```python
from build123d import *

# Parameters (mm, degrees)
SZKIC1_W                    = 100
SZKIC1_H                    = 60
SZKIC1_R                    = 10
DODANIE_WYCI_GNI_CIE1_DEPTH = 15
DODANIE_WYCI_GNI_CIE2_DEPTH = 15
SZKIC3_R                    = 6.5
DODANIE_WYCI_GNI_CIE5_DEPTH = 15


with BuildPart() as part:
    # Szkic1 → Dodanie-wyci_gni_cie1 (new body)
    with BuildSketch(Plane.XY):
        Rectangle(SZKIC1_W, SZKIC1_H)
        Circle(SZKIC1_R, mode=Mode.SUBTRACT)
    extrude(amount=-DODANIE_WYCI_GNI_CIE1_DEPTH)



with BuildPart() as body_2:
    # Szkic2 → Dodanie-wyci_gni_cie2 (new body)
    with BuildSketch(Plane.XY.offset(37)):
        Polygon((-50, 30), (-50, 15), (25, 15), (25, -30), (50, -30), (50, 30), align=None)
    extrude(amount=DODANIE_WYCI_GNI_CIE2_DEPTH)


with BuildPart() as part_1:
    add(part.part)

    add(body_2.part)  # Dodanie-wyci_gni_cie5 merges body 2
    # Szkic3 → Dodanie-wyci_gni_cie5 (add)
    with BuildSketch(Plane(origin=(0, -30, 0), x_dir=(-1, 0, 0), z_dir=(0, -1, 0))):
        Polygon((-25, 0), (-25, -37), (-50, -37), (-50, -15), (-75, -15), (-75, 15), (-50, 15), (-50, 0), align=None)
        with Locations(Location((-63, 0, 0), (0, 0, 90))):
            Circle(SZKIC3_R, mode=Mode.SUBTRACT)
    extrude(amount=-DODANIE_WYCI_GNI_CIE5_DEPTH)


solid = part_1.part
```
Part model, mm, in its own coordinate system. A direction names the side the tool comes from. Round coordinates to 2 decimals unless told otherwise and drop trailing zeros. Order: outer loops, then holes, each group sorted by start corner. A loop starts at its lowest first (then second) coordinate and runs counter-clockwise, first axis right, second up. Notation, with made-up numbers: M 12,-15 L 21,-15 A16 ccw 21,7 Z; hole C -19,-31.5 d11. An arc over 180 degrees is marked long. Answer in a Markdown table with one row per item. Add a question column.
Q1. Wall check: L1, parallel to Z at x = -39, y = 21; L2, parallel to X at y = 9, z = 45; L3, parallel to Y at x = 64, z = 12.5. Give the ranges that are in metal, low to high. Write a range as from..to.
Q2. Mould opens along Z. For faces 6 (the face through (13, 0, -15)), 7 (the face through (1, 30, 44)), 8 (the face through (50, -15, 11)) say: +Z half, -Z half, draft (parallel to the pull), parting line (faces both ways), or undercut.
Q3. Cut at D-D on x = 0. Give the cut face in (y, z), and give its area (3 significant figures).
Q4. Pin check, flat tips, straight feed: pin 1 (8 mm diameter, centred on x = -28, y = -22.5, fed in from +Z); pin 2 (16.5 mm diameter, centred on y = 15, z = -4.5, fed in from +X); pin 3 (4 mm diameter, centred on y = -20.5, z = 6.5, fed in from -X). Stop position of each tip, or through.
Q5. 3-axis set-ups, long thin cutter, end or side, ignore diameter. For faces 1 (the face through (25, -18, 31)), 2 (the face through (10, 18, 37)), 3 (the face through (-12, 0, 0)), 4 (the face through (50, 7, -7)), 5 (the face through (50, -7, 42)): which of +Z, -Z, +X, -X, +Y, -Y reach the whole face in a straight line?
Q6. Cut at C-C on y = 0. Give the cut face in (x, z), and give its area (4 significant figures).
Q7. Cut at A-A on y = 12. Give the cut face in (x, z), and give its area (4 significant figures).
Q8. Cut at B-B on x = 65.5. Give the cut face in (y, z).
Established:
| question | item | result |
|---|---|---|
| 1 | L1 | z = -15..0, 37..52 |
| 1 | L2 | x = 25..50 |
| 1 | L3 | y = -30..-15 |
| 2 | face 6 | -Z half |
| 2 | face 7 | draft |
| 2 | face 8 | undercut |
| 3 | outline | M -30,-15 L -10,-15 L -10,0 L -30,0 Z; M 10,-15 L 30,-15 L 30,0 L 10,0 Z; M 15,37 L 30,37 L 30,52 L 15,52 Z |
| 3 | area | 825 mm2 |
| 4 | pin 1 | stops at z = 0 |
| 4 | pin 2 | stops at x = 50 |
| 4 | pin 3 | stops at x = 25 |
| 5 | face 1 | +Z, -X, -Y |
| 5 | face 2 | +X, -X, +Y |
| 5 | face 3 | -X, +Y |
| 5 | face 4 | +Z, -Z, +X, +Y |
| 5 | face 5 | +Z, +X, +Y, -Y |
| 6 | outline | M -50,-15 L -10,-15 L -10,0 L -50,0 Z; M 10,-15 L 50,-15 L 50,0 L 10,0 Z; M 25,37 L 50,37 L 50,52 L 25,52 Z |
| 6 | area | 1,575 mm2 |
| 7 | outline | M -50,-15 L 50,-15 L 50,0 L -50,0 Z; M 25,37 L 50,37 L 50,52 L 25,52 Z |
| 7 | area | 1,875 mm2 |
| 8 | outline | M -30,-15 L -15,-15 L -15,-6 L -30,-6 Z; M -30,6 L -15,6 L -15,15 L -30,15 Z |
